For this review, use the dimensioned drawing (mm, ordinates from the lowest corner) and the shaded views. Round coordinates to 2 decimals unless told otherwise and drop trailing zeros. Write each loop counter-clockwise with the first axis right and the second up, starting at its lowest first coordinate (ties: lowest second). Pieces come first, ordered by that corner, then holes. Notation, with made-up numbers: M 73.25,35 L 85.25,35 A29 ccw 85.25,72 Z; hole C -24,84 d8. An arc over 180 degrees is marked long. Use CSV: the item, a comma, the result in double quotes.
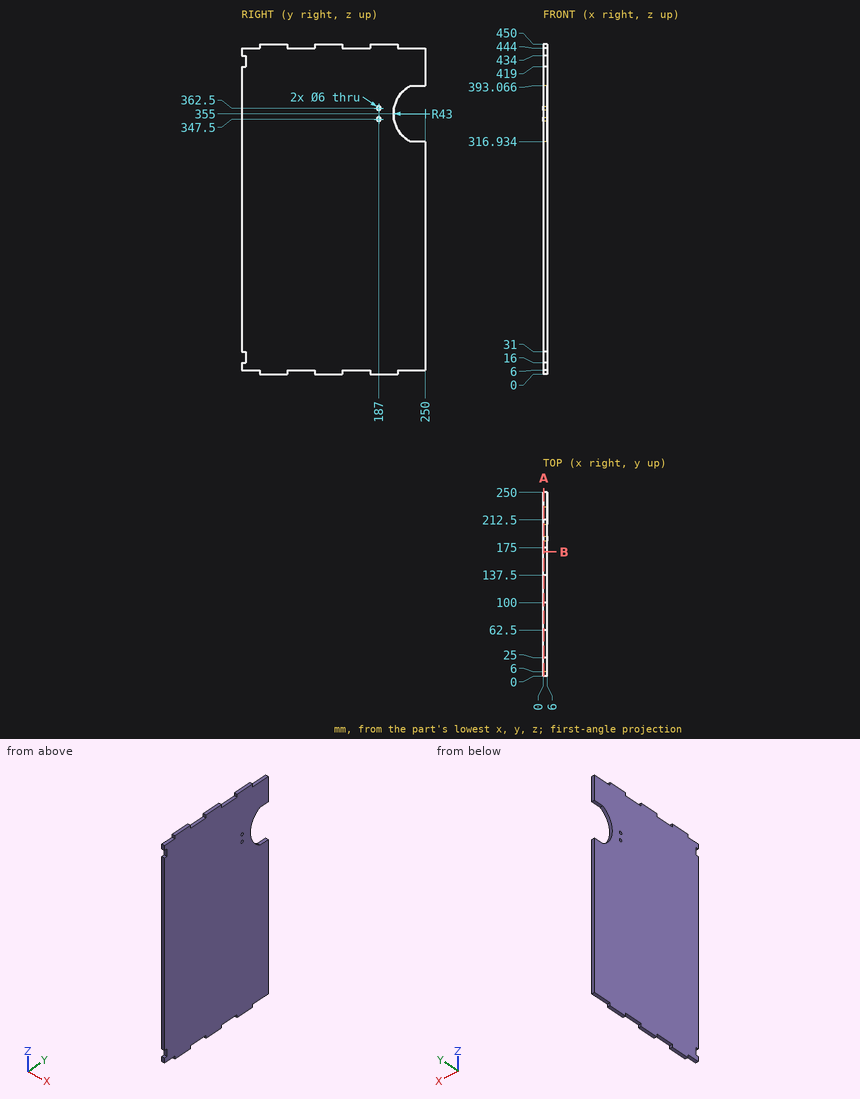
1) Add section A-A on x = 0.95. Give the number of separate pieces and of enclosed holes in the cut face, then the cut area to 3 significant figures.
Answers:
separate pieces,"1"
enclosed holes,"2"
area,"108,000 mm²"
2) Add section B-B on y = 169. Write out the cut boundary in (x, z).
Answers:
outline,"M 0,6 L 6,6 L 6,444 L 0,444 Z"
3) For pin 1 Ø3 at (x, y) = (2, 4.5) entering from -Z; pin 2 Ø3 at (x, z) = (3, 446.5) entering from -Y; pin 3 Ø1.8 at (x, z) = (1.5, 447) entering from +Y, all flat-tipped, find the tip position at first contact; note any pin that passes through.
Answers:
pin 1,"z = 6"
pin 2,"y = 25"
pin 3,"y = 212.5"
4) Wall thickness on line 1 along Z through (x, y) = (4.45, 187); line 2 along Y through (x, z) = (4.15, 362.5); line 3 along Z through (x, y) = (5.5, 12): over which ranges is each line inside the solid? List them lowest first. Write a range as [from, to].
Answers:
line 1,"[0, 344.5], [350.5, 359.5], [365.5, 450]"
line 2,"[0, 184], [190, 207.66]"
line 3,"[6, 444]"
